from build123d import *

# Parameters (mm, degrees)
SKETCH007_R                = 4.2
PAD002_DEPTH               = 1
SKETCH007_MIRRORED003_2_R  = 4.2
PAD002_MIRRORED003_2_DEPTH = 1


with BuildPart() as part:
    # Sketch007 → Pad002 (new body)
    with BuildSketch(Plane(origin=(0, 0, 0), x_dir=(-1, 0, 0), z_dir=(0, 0, -1))):
        with BuildLine():
            ThreePointArc((45.75, 0), (45.637926, 3.20034), (45.302255, 6.385))
            ThreePointArc((45.302255, 6.385), (32.680719, 39.586204), (0, 53.5))
            Line((0, 53.5), (0, 60.5))
            ThreePointArc((49.326147, 54.415147), (24.850021, 58.973043), (0, 60.5))
            ThreePointArc((54.625, 47.624978), (53.143522, 51.931496), (49.326147, 54.415147))
            Line((54.625, 47.624978), (54.625, 0))
            Line((54.625, 0), (45.75, 0))
        make_face()
        with Locations((47.625, 47.625)):
            Circle(SKETCH007_R, mode=Mode.SUBTRACT)
    pad002 = extrude(amount=PAD002_DEPTH)

    # Sketch007 Mirrored003 2 → Pad002 Mirrored003 2 (add)
    with BuildSketch(Plane.XY):
        with BuildLine():
            ThreePointArc((45.75, 0), (45.637926, 3.20034), (45.302255, 6.385))
            ThreePointArc((45.302255, 6.385), (32.680719, 39.586204), (0, 53.5))
            Line((0, 53.5), (0, 60.5))
            ThreePointArc((49.326147, 54.415147), (24.850021, 58.973043), (0, 60.5))
            ThreePointArc((54.625, 47.624978), (53.143522, 51.931496), (49.326147, 54.415147))
            Line((54.625, 47.624978), (54.625, 0))
            Line((54.625, 0), (45.75, 0))
        make_face()
        with Locations((47.625, 47.625)):
            Circle(SKETCH007_MIRRORED003_2_R, mode=Mode.SUBTRACT)
    pad002_mirrored003_2 = extrude(amount=-PAD002_MIRRORED003_2_DEPTH)

    # Mirrored004: Pad002, Pad002 Mirrored003 2 across Sketch007 H_Axis
    add(pad002.mirror(Plane(origin=(0, 0, 0), x_dir=(0, 0, -1), z_dir=(0, 1, 0))))
    add(pad002_mirrored003_2.mirror(Plane(origin=(0, 0, 0), x_dir=(0, 0, -1), z_dir=(0, 1, 0))))


solid = part.part
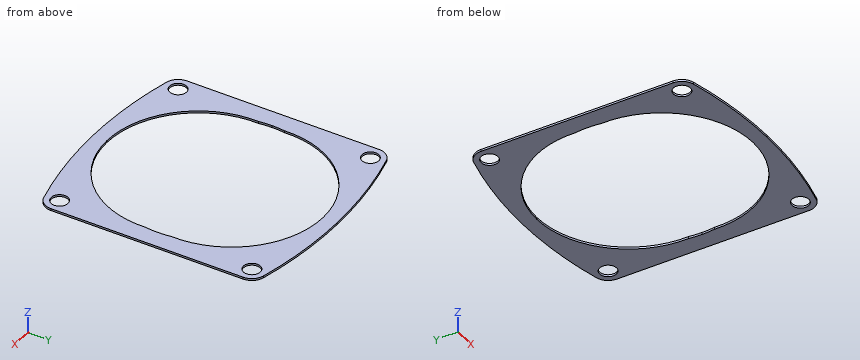
Can you work these out from the model? Positions are in its coordinate system, mm. Round coordinates to 2 decimals unless told otherwise and drop trailing zeros. Write each loop counter-clockwise with the first axis right and the second up, starting at its lowest first coordinate (ties: lowest second). Pieces come first, ordered by that corner, then holes. Notation, with made-up numbers: (-14.5, -16.5) -> (-9.5, -16.5) arc R31 cw to (-9.5, 14.5) -> close; hole circle Ø7 at (1, 69). An arc over 180 degrees is marked (long way). One line per question, with ' | ' between items. Start each with the question number.
1) Suppose I cut it at C-C on y = 50.5. Write out the boundary of the cut face in (x, z), then the cut area to 3 significant figures.
2) Suppose I cut it at D-D on z = -0.55. Count the separate pieces of the cut face and the enclosed holes in it, then the cut area to 3 significant figures.
3) I need wall thicknesses on line 1 (X direction, y = -7.5, z = -0.3) (3 decimals); line 2 (X direction, y = -1.5, z = -0.7) (3 decimals); line 3 (Y direction, x = 1, z = -0.85). Which ranges of each line are inside material? Lowest first, please. Write a range as [from, to].
4) Suppose I cut it at A-A on y = 16. Write out the boundary of the cut face in (x, z) (3 decimals).
5) Suppose I cut it at B-B on x = 2. Write out the boundary of the cut face in (y, z), then the cut area to 3 significant figures.
6) I'm going to push a flat-ended pin straight in: P1, Ø5, axis at x = -47.625, y = -47.625, coming from the -Z side. Where does the tip first touch, or does it pass through?
Return value:
1) outline: (-54.01, -1) -> (-50.69, -1) -> (-50.69, 0) -> (-54.01, 0) -> close; (-44.56, -1) -> (-16.22, -1) -> (-16.22, 0) -> (-44.56, 0) -> close; (16.22, -1) -> (44.56, -1) -> (44.56, 0) -> (16.22, 0) -> close; (50.69, -1) -> (54.01, -1) -> (54.01, 0) -> (50.69, 0) -> close | area: 63.3 mm2
2) separate pieces: 1 | enclosed holes: 5 | area: 4,490 mm2
3) line 1: x = [-54.625, -45.332], [45.332, 54.625] | line 2: x = [-54.625, -45.725], [45.725, 54.625] | line 3: y = [-60.5, -53.49], [53.49, 60.5]
4) outline: (-54.625, -1) -> (-44.655, -1) -> (-44.655, 0) -> (-54.625, 0) -> close; (44.655, -1) -> (54.625, -1) -> (54.625, 0) -> (44.655, 0) -> close
5) outline: (-60.49, -1) -> (-53.46, -1) -> (-53.46, 0) -> (-60.49, 0) -> close; (53.46, -1) -> (60.49, -1) -> (60.49, 0) -> (53.46, 0) -> close | area: 14.1 mm2
6) P1: passes through
